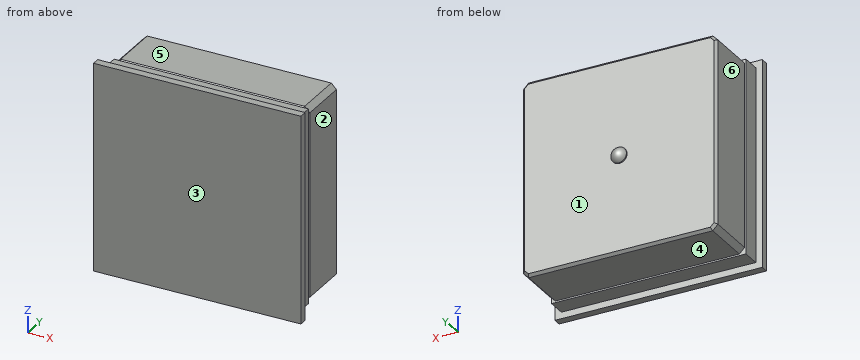
from build123d import *

# Parameters (mm, degrees)
SKETCH1_W           = 16
SKETCH1_H           = 16
BOSS_EXTRUDE1_DEPTH = 0.6
SKETCH2_W           = 15
SKETCH2_H           = 15
BOSS_EXTRUDE2_DEPTH = 1.4
BOSS_EXTRUDE3_DEPTH = 4.2
CHAMFER1_SIZE       = 0.2
SKETCH4_R           = 0.6
BOSS_EXTRUDE4_DEPTH = 0.1
DOME1_FACE_RADIUS   = 0.6
DOME1_HEIGHT        = 0.4


with BuildPart() as part:
    # Sketch1 → Boss-Extrude1 (new body)
    with BuildSketch(Plane(origin=(0, 0, 0), x_dir=(1, 0, 0), z_dir=(0, 1, 0))):
        Rectangle(SKETCH1_W, SKETCH1_H)
    extrude(amount=BOSS_EXTRUDE1_DEPTH)

    # Sketch2 → Boss-Extrude2 (add)
    with BuildSketch(Plane(origin=(0, 0.6, 0), x_dir=(1, 0, 0), z_dir=(0, 1, 0))):
        Rectangle(SKETCH2_W, SKETCH2_H)
    extrude(amount=BOSS_EXTRUDE2_DEPTH)


with BuildPart() as body_2:
    # Sketch3 → Boss-Extrude3 (new body)
    with BuildSketch(Plane(origin=(0, 2, 0), x_dir=(1, 0, 0), z_dir=(0, 1, 0))):
        Polygon((-7.1, 7.5), (-7.5, 7.1), (-7.5, -7.1), (-7.1, -7.5), (7.1, -7.5), (7.5, -7.1), (7.5, 7.1), (7.1, 7.5), align=None)
    extrude(amount=BOSS_EXTRUDE3_DEPTH)

    # Chamfer1
    chamfer1_edges = [body_2.edges().sort_by_distance(p)[0] for p in [
        (0, 6.2, 7.5),
        (-7.3, 2, 7.3),
        (-7.5, 2, 0),
        (7.3, 6.2, 7.3),
        (7.5, 6.2, 0),
        (7.3, 6.2, -7.3),
        (0, 6.2, -7.5),
        (-7.3, 6.2, -7.3),
        (-7.5, 6.2, 0),
        (-7.3, 6.2, 7.3),
        (-7.3, 2, -7.3),
        (0, 2, -7.5),
        (7.3, 2, -7.3),
        (7.5, 2, 0),
        (7.3, 2, 7.3),
        (0, 2, 7.5),
    ]]
    chamfer(chamfer1_edges, length=CHAMFER1_SIZE)

    # Combine1: union part
    add(part.part)

    # Sketch4 → Boss-Extrude4 (add)
    with BuildSketch(Plane(origin=(0, 6.2, 0), x_dir=(1, 0, 0), z_dir=(0, 1, 0))):
        with Locations(Location((0, 0, 0), (0, 0, 270))):
            Circle(SKETCH4_R)
    extrude(amount=BOSS_EXTRUDE4_DEPTH)

    # Dome1: a dome of height H over a round flat face of radius A is a cap of a sphere of radius (A * A + H * H) / (2 * H)
    dome1_r = (DOME1_FACE_RADIUS * DOME1_FACE_RADIUS + DOME1_HEIGHT * DOME1_HEIGHT) / (2 * DOME1_HEIGHT)
    dome1_base = Plane((0, 6.3, 0), z_dir=(0, 1, 0))
    with Locations(dome1_base.offset(DOME1_HEIGHT - dome1_r)):
        dome1_ball = Sphere(dome1_r, mode=Mode.PRIVATE)
    add(split(dome1_ball, bisect_by=dome1_base, keep=Keep.TOP, mode=Mode.PRIVATE))


solid = body_2.part
Could you check a few things on this model? Use its own coordinates, in mm. Face numbers are marked on the shaded views. A direction names the side the tool comes from. Round coordinates to 2 decimals unless told otherwise and drop trailing zeros. Order: outer loops, then holes, each group sorted by start corner. A loop starts at its lowest first (then second) coordinate and runs counter-clockwise, first axis right, second up.
(1) Imagine slicing it at A-A (x = 0). Write out the boundary of the cut face in (y, z).
Response values:
outline: (0, -8) - (0.6, -8) - (0.6, -7.5) - (2, -7.5) - (2, -7.3) - (2.2, -7.5) - (6, -7.5) - (6.2, -7.3) - (6.2, -0.6) - (6.3, -0.6) arc R0.65 ccw to (6.3, 0.6) - (6.2, 0.6) - (6.2, 7.3) - (6, 7.5) - (2.2, 7.5) - (2, 7.3) - (2, 7.5) - (0.6, 7.5) - (0.6, 8) - (0, 8) - close
(2) Which directions (+Z, -Z, +X, -X, +Y, -Y) give clear straight access to the entire face, cutting with the end or side of a thin tool? Please do the marked faces 4, 5 and 6.
Response values:
face 4: -Z, +X, -X, +Y
face 5: +Z, +X, -X, +Y
face 6: +Z, -Z, -X, +Y
(3) Imagine slicing it at D-D (x = -5.75). Write out the boundary of the cut face in (y, z).
Response values:
outline: (0, -8) - (0.6, -8) - (0.6, -7.5) - (2, -7.5) - (2, -7.3) - (2.2, -7.5) - (6, -7.5) - (6.2, -7.3) - (6.2, 7.3) - (6, 7.5) - (2.2, 7.5) - (2, 7.3) - (2, 7.5) - (0.6, 7.5) - (0.6, 8) - (0, 8) - close
(4) If we mould it in two halves opening along Y, with no side actions, what happens to the marked faces 1, 2 and 3? For each: released by +Y, released by -Y, zero draft, split by the parting line, or undercut.
Response values:
face 1: released by +Y
face 2: zero draft
face 3: released by -Y
(5) Please list where these lines run through material, in increasing order: line 1 along Z through (x, y) = (-4, 4.5); line 2 along Y through (x, z) = (-3.75, 0.5).
Response values:
line 1: z = -7.5 to 7.5
line 2: y = 0 to 6.2
(6) Imagine slicing it at B-B (z = 1.25). Write out the boundary of the cut face in (x, y).
Response values:
outline: (-8, 0) - (8, 0) - (8, 0.6) - (7.5, 0.6) - (7.5, 2) - (7.3, 2) - (7.5, 2.2) - (7.5, 6) - (7.3, 6.2) - (-7.3, 6.2) - (-7.5, 6) - (-7.5, 2.2) - (-7.3, 2) - (-7.5, 2) - (-7.5, 0.6) - (-8, 0.6) - close
(7) I'm going to push flat-ended pins straight in: pin 1 (0.7 mm diameter, centred on y = 1, z = -0.5, fed in from +X); pin 2 (4 mm diameter, centred on x = 0, y = 3.5, fed in from +Z); pin 3 (1.5 mm diameter, centred on y = 1.5, z = -2.5, fed in from -X). Where does each tip first touch, or does it pass through?
Response values:
pin 1: stops at x = 7.5
pin 2: stops at z = 7.5
pin 3: stops at x = -7.5
(8) Imagine slicing it at C-C (y = 3.25). Write out the boundary of the cut face in (x, z).
Response values:
outline: (-7.5, -7.1) - (-7.1, -7.5) - (7.1, -7.5) - (7.5, -7.1) - (7.5, 7.1) - (7.1, 7.5) - (-7.1, 7.5) - (-7.5, 7.1) - close
